```python
from build123d import *

# Parameters (mm, degrees)
SKETCH1_W                 = 65
SKETCH1_H                 = 26
BOSS_EXTRUDE1_DEPTH       = 4
F_2_5MM_DOWEL_HOLE1_D     = 2.5
F_2_5MM_DOWEL_HOLE1_DEPTH = 5
F_2_5MM_DOWEL_HOLE1_TIP   = 0.751075774
SKETCH6_W                 = 65
SKETCH6_H                 = 26
BOSS_EXTRUDE2_DEPTH       = 20
BOSS_EXTRUDE2_TAPER       = 7
SKETCH7_W                 = 48.088617564
SKETCH7_H                 = 13.088617564
CUT_EXTRUDE1_DEPTH        = 20
CUT_EXTRUDE1_DRAFT        = 7
CUT_EXTRUDE3_DEPTH        = 33
CUT_EXTRUDE4_DEPTH        = 70
SKETCH11_W                = 60.088617564
SKETCH11_H                = 21.088617564
BOSS_EXTRUDE3_DEPTH       = 6
SKETCH12_W                = 60.088617564
SKETCH12_H                = 21.088617564
BOSS_EXTRUDE5_DEPTH       = 70
BOSS_EXTRUDE5_TAPER       = 4
CUT_EXTRUDE5_DEPTH        = 55
CUT_EXTRUDE6_DEPTH        = 67
F_2_5MM_DOWEL_HOLE2_D     = 2.5
F_2_5MM_DOWEL_HOLE2_DEPTH = 5
F_2_5MM_DOWEL_HOLE2_TIP   = 0.751075774


with BuildPart() as part:
    # Sketch1 → Boss-Extrude1 (new body)
    with BuildSketch(Plane(origin=(0, 0, 0), x_dir=(1, 0, 0), z_dir=(0, 1, 0))):
        with Locations((32.5, 13)):
            Rectangle(SKETCH1_W, SKETCH1_H)
    extrude(amount=BOSS_EXTRUDE1_DEPTH)

    # Ø2.5mm Dowel Hole1
    with Locations(Plane(origin=(23.5, 4, -13), x_dir=(0, 0, 1), z_dir=(0, 1, 0))):
        with Locations((0, 0), (-6.92820323, 12), (6.92820323, 12)):
            Hole(F_2_5MM_DOWEL_HOLE1_D / 2, depth=F_2_5MM_DOWEL_HOLE1_DEPTH)
            with Locations((0, 0, -(F_2_5MM_DOWEL_HOLE1_DEPTH + F_2_5MM_DOWEL_HOLE1_TIP / 2))):  # 118° drill point
                Cone(0, F_2_5MM_DOWEL_HOLE1_D / 2, F_2_5MM_DOWEL_HOLE1_TIP, mode=Mode.SUBTRACT)

    # Sketch6 → Boss-Extrude2 (add)
    with BuildSketch(Plane(origin=(0, 4, 0), x_dir=(1, 0, 0), z_dir=(0, 1, 0))):
        with Locations((32.5, 13)):
            Rectangle(SKETCH6_W, SKETCH6_H)
    extrude(amount=BOSS_EXTRUDE2_DEPTH, taper=BOSS_EXTRUDE2_TAPER)


with BuildPart() as cut_extrude1_tool:
    # Sketch7 → Cut-Extrude1 (with draft: the straight prism first)
    with BuildSketch(Plane(origin=(0, 24, 0), x_dir=(1, 0, 0), z_dir=(0, 1, 0))):
        with Locations((32.5, 13)):
            Rectangle(SKETCH7_W, SKETCH7_H)
    extrude(amount=-CUT_EXTRUDE1_DEPTH)
    # Cut-Extrude1: the draft: its side faces are tilted about the plane it starts from
    cut_extrude1_sides = [cut_extrude1_tool.faces().sort_by_distance(p)[0] for p in [
        (8.455691218, 14, -13),
        (32.5, 14, -6.455691218),
        (56.544308782, 14, -13),
        (32.5, 14, -19.544308782),
    ]]
    draft(cut_extrude1_sides, Plane(origin=(0, 24, 0), x_dir=(1, 0, 0), z_dir=(0, 1, 0)), CUT_EXTRUDE1_DRAFT)


with BuildPart() as part_1:
    add(part.part)

    # Cut-Extrude1: cut by cut_extrude1_tool
    add(cut_extrude1_tool.part, mode=Mode.SUBTRACT)

    # Sketch9 → Cut-Extrude3 (cut)
    with BuildSketch(Plane(origin=(0, 0, -26), x_dir=(-1, 0, 0), z_dir=(0, 0, -1))):
        Polygon((-59, 4), (-6, 4), (-8.455691218, 24), (-56.544308782, 24), align=None)
    extrude(amount=-CUT_EXTRUDE3_DEPTH, mode=Mode.SUBTRACT)

    # Sketch10 → Cut-Extrude4 (cut)
    with BuildSketch(Plane(origin=(65, 0, 0), x_dir=(0, 0, -1), z_dir=(1, 0, 0))):
        Polygon((4, 4), (22, 4), (19.544308782, 24), (6.455691218, 24), align=None)
    extrude(amount=-CUT_EXTRUDE4_DEPTH, mode=Mode.SUBTRACT)

    # Sketch11 → Boss-Extrude3 (add)
    with BuildSketch(Plane(origin=(0, 24, 0), x_dir=(1, 0, 0), z_dir=(0, 1, 0))):
        with Locations((32.5, 13)):
            Rectangle(SKETCH11_W, SKETCH11_H)
    extrude(amount=BOSS_EXTRUDE3_DEPTH)

    # Sketch12 → Boss-Extrude5 (add)
    with BuildSketch(Plane(origin=(0, 30, 0), x_dir=(1, 0, 0), z_dir=(0, 1, 0))):
        with Locations((32.5, 13)):
            Rectangle(SKETCH12_W, SKETCH12_H)
    extrude(amount=BOSS_EXTRUDE5_DEPTH, taper=BOSS_EXTRUDE5_TAPER)

    # Sketch13 → Cut-Extrude5 (cut)
    with BuildSketch(Plane(origin=(0, 0, -23.544308782), x_dir=(-1, 0, 0), z_dir=(0, 0, -1))):
        Polygon((-62.544308782, 30), (-43.787865312, 100), (-62.544308782, 100), align=None)
        Polygon((-2.455691218, 30), (-21.212134688, 100), (-2.455691218, 100), align=None)
        Polygon((-39.049928788, 94.5), (-25.950071212, 94.5), (-8.455691218, 30), (-56.544308782, 30), align=None)
    extrude(amount=-CUT_EXTRUDE5_DEPTH, mode=Mode.SUBTRACT)

    # Sketch14 → Cut-Extrude6 (cut)
    with BuildSketch(Plane(origin=(62.544308782, 0, 0), x_dir=(0, 0, -1), z_dir=(1, 0, 0))):
        Polygon((6.455691218, 30), (19.986565131, 30), (15.024261819, 94.5), (10.965970588, 94.5), align=None)
    extrude(amount=-CUT_EXTRUDE6_DEPTH, mode=Mode.SUBTRACT)

    # Ø2.5mm Dowel Hole2
    with Locations(Plane(origin=(0, 100, 0), x_dir=(1, 0, 0), z_dir=(0, 1, 0))):
        with Locations((28.5, 13), (36.5, 13)):
            Hole(F_2_5MM_DOWEL_HOLE2_D / 2, depth=F_2_5MM_DOWEL_HOLE2_DEPTH)
            with Locations((0, 0, -(F_2_5MM_DOWEL_HOLE2_DEPTH + F_2_5MM_DOWEL_HOLE2_TIP / 2))):  # 118° drill point
                Cone(0, F_2_5MM_DOWEL_HOLE2_D / 2, F_2_5MM_DOWEL_HOLE2_TIP, mode=Mode.SUBTRACT)


solid = part_1.part
```
The listing builds one solid part. Answer for the finished solid, in the listing's coordinates (mm). A direction names the side the tool comes from. Round coordinates to 2 decimals unless told otherwise and drop trailing zeros. Use CSV: the item, a comma, the result in double quotes. Start each with the question number.
(1) Consider L1, parallel to Y at x = 43, z = -13; L2, parallel to Z at x = 35, y = 1; L3, parallel to Y at x = 52, z = -12. Determine where each line is inside the solid, lowest interval first. Write a range as from..to.
(2) Which of the six approach directions +Z, -Z, +X, -X, +Y, -Y give full straight-line access (tool end or side, diameter ignored) to faces 4 (the face through (51.722, 62.1, -17.517)), 5 (the face through (34.28, 1.97, -5.8)), 6 (the face through (7.21, 13.86, -22.82)), 7 (the face through (33, 94.5, -13))?
(3) Each of these flat-tipped pins is pushed along its axis until it touches: pin 1 (3 mm diameter, centred on x = 24.5, y = 30, fed in from -Z); pin 2 (12 mm diameter, centred on x = 29, y = 62, fed in from -Z); pin 3 (9.5 mm diameter, centred on x = 37, z = -12, fed in from -Y); pin 4 (5 mm diameter, centred on x = 30, y = 26, fed in from +Z). Where does it stop, or does it pass through?
(4) The mould has two halves that part along Z. Classify faces 1 (the face through (57.755, 14.14, -22.817)), 2 (the face through (32, 2, -26)), 3 (the face through (50.85, 62.4, -8.72)): released by +Z, released by -Z, zero draft, split by the parting line, or undercut.
(5) Section A-A on y = 33 is taken. Count the separate pieces of the cut face and the enclosed holes in it, then the cut area to 3 significant figures.
A:
1,L1,"y = 0..4, 24..30, 94.5..100"
1,L2,"z = -26..-21.07, -18.78..-7.22, -4.93..0"
1,L3,"y = 0..4, 24..30"
2,face 4,"+X, -X"
2,face 5,"-Y"
2,face 6,"+Z, -Z"
2,face 7,"none"
3,pin 1,"stops at z = -23.54"
3,pin 2,"passes through"
3,pin 3,"stops at y = 0"
3,pin 4,"stops at z = -2.46"
4,face 1,"zero draft"
4,face 2,"released by -Z"
4,face 3,"undercut"
5,separate pieces,"4"
5,enclosed holes,"0"
5,area,"91.1 mm²"
